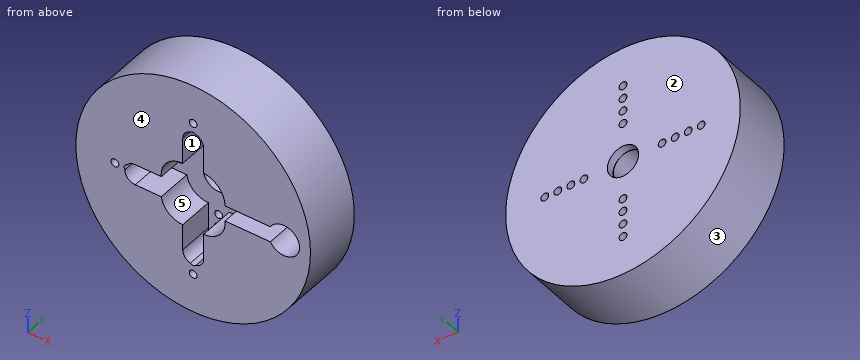
Solid Edge part; units mm, degrees
sketch "Sketch1" plane through (0, 0, 0) normal (0, -1, 0) x (1, 0, 0)
  circle A0 centre (80.5127, 55.3877) radius 22.5
extrude "Protrusion1" add sketch "Sketch1" against normal blind 10
sketch "Sketch2" plane through (80.5127, 10, 55.3877) normal (0, 1, 0) x (0, 0, -1)
  circle A0 centre (0, 0) radius 2.95
extrude "ExtrudedCutout_5" cut sketch "Sketch2" against normal blind 4
sketch "Sketch3" plane through (80.5127, 6, 55.3877) normal (0, 1, 0) x (-1, 0, 0)
  circle A0 centre (0, 0) radius 1.05
extrude "Cutout1" cut sketch "Sketch3" against normal up to next
sketch "Sketch4" plane through (80.5127, 5, 51.1598) normal (0, -1, 0) x (1, 0, 0)
  circle A0 centre (0, 4.2279) radius 3.55
extrude "ExtrudedCutout_7" cut sketch "Sketch4" against normal blind 0.5
chamfer "Chamfer_2" distance 1.9 distance2 0.5 1 edges at (80.5127, 6, 58.3377) measured on face at (78.605, 6, 53.362)
sketch "Sketch5" plane through (80.5127, 10, 55.3877) normal (0, 1, 0) x (0, 0, 1)
  circle A0 centre (0, 0) radius 22.5
  circle A1 centre (0, 0) radius 3
extrude "ExtrudedProtrusion_4" add sketch "Sketch5" along normal blind 1.5
sketch "Sketch6" plane through (80.5127, 0, 55.3877) normal (0, -1, 0) x (0, 0, 1)
  line L0 (1.5, 11.11) -> (1.5, 6.11)
  arc A0 (6.11, 2) -> (1.5, 6.11) centre (1.9729, 2) ccw
  line L1 (6.11, 2) -> (11.11, 2)
  arc A1 (11.11, 2) -> (11.11, -2) centre (11.11, 0) cw
  line L2 (11.11, -2) -> (6.11, -2)
  arc A2 (1.4978, -6.11) -> (6.11, -2) centre (1.4978, -1.4671) ccw
  line L3 (1.4978, -14.81) -> (1.4978, -6.11)
  arc A3 (-1.5, -14.81) -> (1.4978, -14.81) centre (-0.0011, -17.4087) ccw
  line L4 (-1.5, -6.11) -> (-1.5, -14.81)
  arc A4 (-6.11, -2) -> (-1.5, -6.11) centre (-1.9729, -2) ccw
  line L5 (-11.11, -2) -> (-6.11, -2)
  arc A5 (-11.11, 2) -> (-11.11, -2) centre (-11.11, 0) ccw
  line L6 (-6.11, 2) -> (-11.11, 2)
  arc A6 (-6.11, 2) -> (-2.5, 6.11) centre (-1.9654, 2) cw
  line L7 (-2.5, 11.11) -> (-2.5, 6.11)
  arc A7 (1.5, 11.11) -> (-2.5, 11.11) centre (-0.5, 11.11) ccw
  dimension "D1" = 1.5
  dimension "D2" = 2.5
  dimension "D3" = 6.11
  dimension "D4" = 11.11
  dimension "D5" = 6.11
  dimension "D6" = 1.5
  dimension "D7" = 1.4978
  dimension "D8" = 11.11
extrude "ExtrudedCutout_9" cut sketch "Sketch6" against normal blind 6.7
sketch "Sketch7" plane through (80.5127, 11.5, 55.3877) normal (0, 1, 0) x (0, 0, -1)
  circle A0 centre (7.5, 0) radius 0.75
  circle A1 centre (10, 0) radius 0.75
  circle A2 centre (12.5, 0) radius 0.75
  circle A3 centre (15, 0) radius 0.75
  circle A4 centre (-15, 0) radius 0.75
  circle A5 centre (-12.5, 0) radius 0.75
  circle A6 centre (-10, 0) radius 0.75
  circle A7 centre (-7.5, 0) radius 0.75
  circle A8 centre (0, -10) radius 0.75
  circle A9 centre (0, -12.5) radius 0.75
  circle A10 centre (0, -15) radius 0.75
  circle A11 centre (0, -7.5) radius 0.75
  circle A12 centre (0, 7.5) radius 0.75
  circle A13 centre (0, 10) radius 0.75
  circle A14 centre (0, 12.5) radius 0.75
  circle A15 centre (0, 15) radius 0.75
extrude "Cutout2" cut sketch "Sketch7" against normal through all
For this review, take the finished solid that the model builds, in its own axes (mm). Face numbers are marked on the shaded views. A direction names the side the tool comes from. Give positions to 0.01 mm unless a question says otherwise; leave off trailing zeros. Loops run counter-clockwise (first coordinate to the right, second up) from the corner with the lowest first, then second, coordinate; pieces in that order, holes last. Notation, with made-up numbers: M 55.5,-10.5 L 66.5,-10.5 A19 cw 66.5,-0.5 Z; hole C -18.75,-3.5 d4. An arc over 180 degrees is marked long. One line per item, written item: value. Start each with the question number.
Q1. Add section A-A (y = 5.25). Give the boundary of the cut face in (x, z).
Q2. Add section D-D (y = 9.25). Count the separate pieces of the cut face and the enclosed holes in it, and give its area (3 significant figures).
Q3. Add section C-C (x = 86). Give the boundary of the cut face in (y, z), and give its area (3 significant figures).
Q4. Clearance check with flat-ended pins moving along their axes: pin 1 Ø1.5 at (y, z) = (5.5, 60.5) entering from -X; pin 2 Ø1.5 at (y, z) = (6, 70.5) entering from +X; pin 3 Ø2 at (y, z) = (4.5, 68) entering from -X. State where each tip first meets the part, or that it passes through.
Q5. For L1, parallel to Z at x = 68.5, y = 8; L2, parallel to Z at x = 68, y = 6.75; L3, parallel to X at y = 4.75, z = 65, list the stretches that pass through material, from the lowest coordinate up.
Q6. Machinability: for the marked faces 1 and 2, which of the approach directions +Z, -Z, +X, -X, +Y, -Y give a long, thin tool a straight path to every point of the face, cutting with its end or side? Answer none if there is none.
Q7. Add section B-B (z = 40.5). Give the boundary of the cut face in (x, y).
Q8. Draft analysis for pull direction Z (two halves, no side actions). For the marked faces 3, 4 and 5, state which applies: released by +Z, released by -Z, zero draft, split by the parting line, or undercut.
Reply:
1. outline: C 80.51,55.39 d45; hole C 65.51,55.39 d1.5; hole M 67.4,54.95 A2 ccw 69.4,52.89 L 74.4,52.89 A4.14 ccw 78.51,49.28 L 78.51,44.28 A2 ccw 79.99,42.35 A0.75 ccw 81.03,42.35 A2 ccw 82.51,44.28 L 82.51,49.28 A4.14 ccw 86.62,53.89 L 95.32,53.89 A3 ccw long 95.32,56.89 L 86.62,56.89 A4.64 ccw 82.51,61.5 L 82.51,66.5 A2 ccw 81.03,68.43 A0.75 ccw 79.99,68.43 A2 ccw 78.51,66.5 L 78.51,61.5 A4.14 ccw 74.4,56.89 L 69.4,56.89 A2 ccw 67.82,56.11 A0.75 ccw Z; hole C 80.51,40.39 d1.5; hole C 80.51,70.39 d1.5
2. separate pieces: 1
2. enclosed holes: 17
2. area: 1,530 mm²
3. outline: M 0,33.57 L 11.5,33.57 L 11.5,77.21 L 0,77.21 L 0,59.21 L 6.7,59.21 L 6.7,51.19 L 0,51.19 Z
3. area: 448 mm²
4. pin 1: x = 58.44
4. pin 2: x = 97.83
4. pin 3: x = 61.24
5. L1: 36.36 to 54.82, 55.96 to 74.41
5. L2: 36.69 to 54.64, 56.14 to 74.09
5. L3: 60.17 to 78.51, 82.51 to 100.86
6. face 1: -Y
6. face 2: +Z, -Z, +X, -X, +Y
7. outline: M 63.64,0 L 79.77,0 L 79.77,11.5 L 63.64,11.5 Z; M 81.25,0 L 97.38,0 L 97.38,11.5 L 81.25,11.5 Z
8. face 3: split by the parting line
8. face 4: zero draft
8. face 5: undercut
